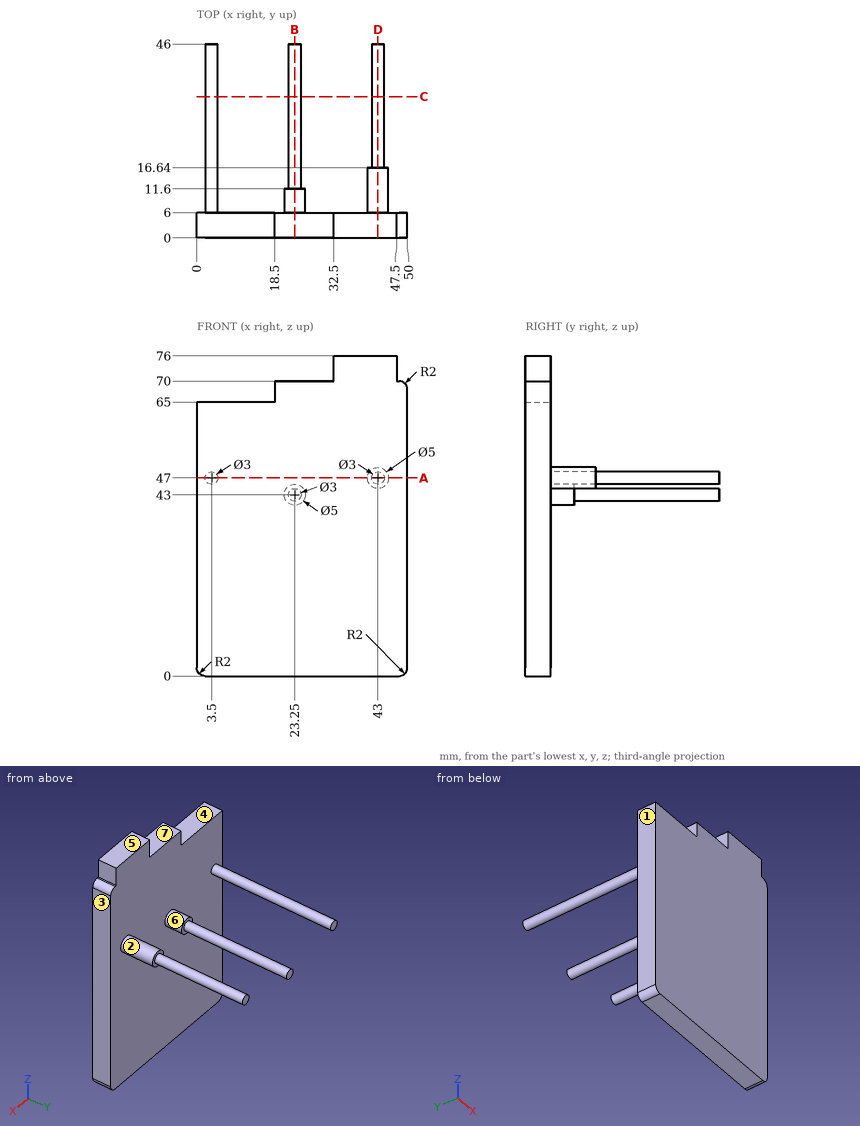
The figure shows three views and two pictorial views of one solid part (mm, origin at its lowest corner). Answer the questions. A direction names the side the tool comes from. Round coordinates to 2 decimals unless told otherwise and drop trailing zeros. Order: outer loops, then holes, each group sorted by start corner. A loop starts at its lowest first (then second) coordinate and runs counter-clockwise, first axis right, second up. Notation, with made-up numbers: (-22.75, 70.25) -> (9.25, 70.25) arc R22 ccw to (9.25, 98.25) -> close; hole circle Ø5 at (26.5, 41). An arc over 180 degrees is marked (long way). One line per item, written item: value.
Item 1: Given P1, Ø6.5, axis at y = 4, z = 72, coming from the -X side; P2, Ø2, axis at x = 44.5, z = 55, coming from the +Y side; P3, Ø3, axis at x = 13.5, y = 3.5, coming from the +Z side; P4, Ø8, axis at x = 30, z = 58.5, coming from the -Y side, each flat-ended and moving along its own axis, determine where each tip first touches the part or whether it passes through.
Taken from the geometry:
P1: stops at x = 18.5
P2: stops at y = 6
P3: stops at z = 65
P4: stops at y = 0
Item 2: For the marked faces 5, 6 and 7, determine the directions among +Z, -Z, +X, -X, +Y, -Y from which every point of the face is accessible in a straight line to the end or side of a thin tool.
Taken from the geometry:
face 5: +Z, +X, -X, +Y, -Y
face 6: +Y
face 7: +Z, -X, +Y, -Y
Item 3: Straight lines are drawn through the part: L1, parallel to Z at x = 13, y = 5; L2, parallel to Y at x = 46, z = 42; L3, parallel to X at y = 6.5, z = 43.5. For each, find the intervals that lie inside material, in ascending order.
Taken from the geometry:
L1: z = 0 to 65
L2: y = 0 to 6
L3: x = 20.8 to 25.7
Item 4: For a pull along X with two mould halves and no side action, classify the marked faces 1, 2, 3 and 4 as released by +X, released by -X, zero draft, split by the parting line, or undercut.
Taken from the geometry:
face 1: released by -X
face 2: undercut
face 3: released by +X
face 4: zero draft
Item 5: Find section C-C, the plane y = 33.5. Give the vertices of the cut face in (x, z), then the cut area to 3 significant figures.
Taken from the geometry:
outline: circle Ø3 at (3.5, 47); circle Ø3 at (23.25, 43); circle Ø3 at (43, 47)
area: 21.2 mm2
Item 6: Find section B-B, the plane x = 23.25. Give the vertices of the cut face in (y, z), then the cut area to 3 significant figures.
Taken from the geometry:
outline: (0, 0) -> (6, 0) -> (6, 40.5) -> (11.6, 40.5) -> (11.6, 41.5) -> (46, 41.5) -> (46, 44.5) -> (11.6, 44.5) -> (11.6, 45.5) -> (6, 45.5) -> (6, 70) -> (0, 70) -> close
area: 551 mm2
Item 7: Find section D-D, the plane x = 43. Give the vertices of the cut face in (y, z), then the cut area to 3 significant figures.
Taken from the geometry:
outline: (0, 0) -> (6, 0) -> (6, 44.5) -> (16.64, 44.5) -> (16.64, 45.5) -> (46, 45.5) -> (46, 48.5) -> (16.64, 48.5) -> (16.64, 49.5) -> (6, 49.5) -> (6, 76) -> (0, 76) -> close
area: 597 mm2
Item 8: Find section A-A, the plane z = 47. Give the vertices of the cut face in (x, y), then the cut area to 3 significant figures.
Taken from the geometry:
outline: (0, 0) -> (50, 0) -> (50, 6) -> (45.5, 6) -> (45.5, 16.64) -> (44.5, 16.64) -> (44.5, 46) -> (41.5, 46) -> (41.5, 16.64) -> (40.5, 16.64) -> (40.5, 6) -> (5, 6) -> (5, 46) -> (2, 46) -> (2, 6) -> (0, 6) -> close
area: 561 mm2
